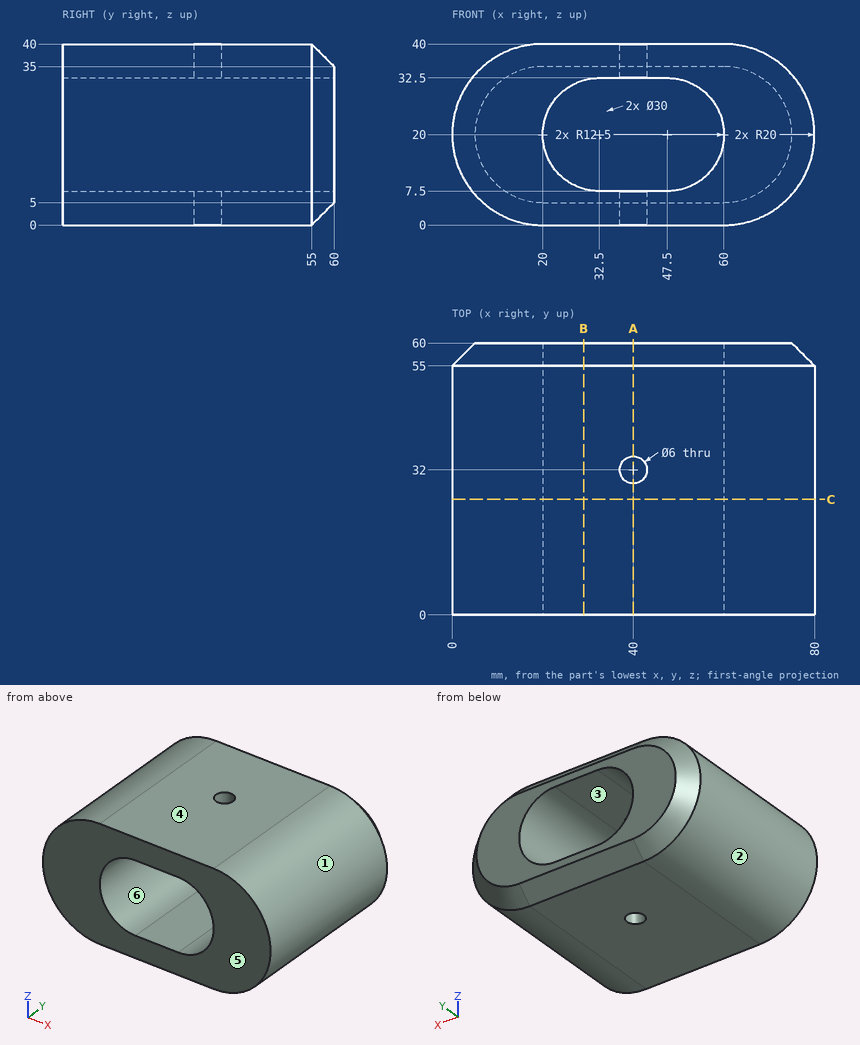
Input: dimensioned drawing with shaded views. Units: mm. Origin: part minimum x, y, z. A direction names the side the tool comes from. Give positions to 0.01 mm unless a question says otherwise; leave off trailing zeros. Order: outer loops, then holes, each group sorted by start corner. A loop starts at its lowest first (then second) coordinate and runs counter-clockwise, first axis right, second up.
(1) Material intervals for line 1 along Z through (x, y) = (43.5, 31); line 2 along Y through (x, z) = (40, 34); line 3 along X through (y, z) = (14.5, 8.5), sorted ascending.
(2) Access query for the marked faces 5 and 6. Directions: +Z, -Z, +X, -X, +Y, -Y. A direction counts if a zero-diameter tool reaches every point of the face in a straight line with its end or side. Return the directions, or none.
(3) Section query C-C (y = 25.5). Return the cut outline in (x, z), plus the area to 3 significant figures.
(4) Section query A-A (x = 40). Return the cut outline in (y, z), plus the area to 3 significant figures.
(5) Pull-direction query (X, two-part tool) for the marked faces 1, 2, 3 and 4; classes: +X half, -X half, draft (parallel to the pull), parting line (faces both ways), or undercut.
(6) Section query B-B (x = 29). Return the cut outline in (y, z).
(7) Contact query for flat-ended pins moving along their axis: P1, Ø6, axis at y = 47.5, z = 21, coming from the -X side; P2, Ø8, axis at x = 65, y = 46, coming from the -Z side (3 decimals); P3, Ø5, axis at x = 67.5, y = 12.5, coming from the +Z side. Output: stop coordinate, or through.
Outcome:
1. line 1: z = 0 to 7.5, 32.5 to 40
1. line 2: y = 0 to 29, 35 to 60
1. line 3: x = 3.64 to 27.6, 52.4 to 76.36
2. face 5: +Z, -Z, +X, -X, -Y
2. face 6: +Y, -Y
3. outline: (20, 0) - (60, 0) arc R20 ccw to (60, 40) - (20, 40) arc R20 ccw to start; hole (32.5, 7.5) - (47.5, 7.5) arc R12.5 ccw to (47.5, 32.5) - (32.5, 32.5) arc R12.5 ccw to start
3. area: 1,990 mm2
4. outline: (0, 0) - (29, 0) - (29, 7.5) - (0, 7.5) - close; (0, 32.5) - (29, 32.5) - (29, 40) - (0, 40) - close; (35, 0) - (55, 0) - (60, 5) - (60, 7.5) - (35, 7.5) - close; (35, 32.5) - (60, 32.5) - (60, 35) - (55, 40) - (35, 40) - close
4. area: 785 mm2
5. face 1: +X half
5. face 2: -X half
5. face 3: undercut
5. face 4: draft
6. outline: (0, 0) - (55, 0) - (60, 5) - (60, 8) - (0, 8) - close; (0, 32) - (60, 32) - (60, 35) - (55, 40) - (0, 40) - close
7. P1: stops at x = 0
7. P2: stops at z = 0.025
7. P3: stops at z = 39.36
